from build123d import *

# Parameters (mm, degrees)
SKETCH1_W           = 280
SKETCH1_H           = 215
BOSS_EXTRUDE1_DEPTH = 10.6
FILLET1_R           = 18
CUT_EXTRUDE1_DEPTH  = 177.829324491
SKETCH3_R           = 1.6
SKETCH3_R_2         = 3.15
SKETCH3_R_3         = 1.7
SKETCH3_R_4         = 1.55
SKETCH3_R_5         = 2
CUT_EXTRUDE2_DEPTH  = 177.829324491


with BuildPart() as part:
    # Sketch1 → Boss-Extrude1 (new body)
    with BuildSketch(Plane(origin=(0, 0, 0), x_dir=(1, 0, 0), z_dir=(0, 1, 0))):
        Rectangle(SKETCH1_W, SKETCH1_H)
    extrude(amount=BOSS_EXTRUDE1_DEPTH)

    # Fillet1
    fillet1_edges = [part.edges().sort_by_distance(p)[0] for p in [
        (-140, 5.3, -107.5),
        (140, 5.3, -107.5),
        (140, 5.3, 107.5),
        (-140, 5.3, 107.5),
    ]]
    fillet(fillet1_edges, radius=FILLET1_R)

    # Sketch2 → Cut-Extrude1 (cut, through all)
    with BuildSketch(Plane(origin=(0, 10.6, 0), x_dir=(1, 0, 0), z_dir=(0, 1, 0))):
        with BuildLine():
            Line((-123.3, -36.5), (-123.3, 36.5))
            ThreePointArc((-123.3, 36.5), (-113.3, 46.5), (-103.3, 36.5))
            Line((-103.3, 36.5), (-103.3, -36.5))
            ThreePointArc((-103.3, -36.5), (-113.3, -46.5), (-123.3, -36.5))
        make_face()
    extrude(amount=-CUT_EXTRUDE1_DEPTH, mode=Mode.SUBTRACT)

    # Sketch3 → Cut-Extrude2 (cut, through all)
    with BuildSketch(Plane(origin=(0, 10.6, 0), x_dir=(1, 0, 0), z_dir=(0, 1, 0))):
        with Locations(Location((-131.75, -27.9, 0), (0, 0, 270))):
            Circle(SKETCH3_R)
        with Locations(Location((-131.75, 30.1, 0), (0, 0, 270))):
            Circle(SKETCH3_R)
        with Locations(Location((-70.6, 20, 0), (0, 0, 270))):
            Circle(SKETCH3_R_2)
        with Locations(Location((-70.6, 0, 0), (0, 0, 270))):
            Circle(SKETCH3_R_3)
        with Locations(Location((-28.3, -10.442748969, 0), (0, 0, 270))):
            Circle(SKETCH3_R)
        with Locations(Location((-37.3, -10.442748969, 0), (0, 0, 270))):
            Circle(SKETCH3_R)
        with Locations(Location((-37.3, 2.5, 0), (0, 0, 270))):
            Circle(SKETCH3_R_4)
        with Locations(Location((-37.3, 20, 0), (0, 0, 270))):
            Circle(SKETCH3_R)
        with Locations(Location((-37.3, 37.5, 0), (0, 0, 270))):
            Circle(SKETCH3_R_4)
        with Locations(Location((-28.3, 50.442748969, 0), (0, 0, 270))):
            Circle(SKETCH3_R)
        with Locations(Location((-37.3, 50.442748969, 0), (0, 0, 270))):
            Circle(SKETCH3_R)
        with Locations(Location((46.6, -4.8, 0), (0, 0, 270))):
            Circle(SKETCH3_R)
        with Locations(Location((46.6, 44.8, 0), (0, 0, 270))):
            Circle(SKETCH3_R)
        with Locations(Location((-70.6, 39.2, 0), (0, 0, 270))):
            Circle(SKETCH3_R_3)
        with Locations(Location((53.7, 44.8, 0), (0, 0, 270))):
            Circle(SKETCH3_R)
        with Locations(Location((53.7, -4.8, 0), (0, 0, 270))):
            Circle(SKETCH3_R)
        with Locations(Location((-39.5, -35, 0), (0, 0, 270))):
            Circle(SKETCH3_R_5)
        with Locations(Location((-14.5, -35, 0), (0, 0, 270))):
            Circle(SKETCH3_R_5)
        with Locations(Location((-39.5, -65, 0), (0, 0, 270))):
            Circle(SKETCH3_R_5)
        with Locations(Location((-14.5, -65, 0), (0, 0, 270))):
            Circle(SKETCH3_R_5)
        with Locations(Location((94.5, -35, 0), (0, 0, 270))):
            Circle(SKETCH3_R_5)
        with Locations(Location((119.5, -35, 0), (0, 0, 270))):
            Circle(SKETCH3_R_5)
        with Locations(Location((94.5, -65, 0), (0, 0, 270))):
            Circle(SKETCH3_R_5)
        with Locations(Location((119.5, -65, 0), (0, 0, 270))):
            Circle(SKETCH3_R_5)
    extrude(amount=-CUT_EXTRUDE2_DEPTH, mode=Mode.SUBTRACT)


solid = part.part
Read the model definition and answer for the solid it produces. Units are mm, in the model's axes. A direction names the side the tool comes from. Coordinates: 2 decimals unless noted, no trailing zeros. Loops run counter-clockwise (first coordinate to the right, second up) from the corner with the lowest first, then second, coordinate; pieces in that order, holes last. Notation, with made-up numbers: (55, 54.5) - (87, 54.5) arc R17 cw to (87, 82.5) - close; hole circle Ø5 at (31, 74). An arc over 180 degrees is marked (long way). Answer in a Markdown table with one row per item.
Q1. Find section C-C on y = 4.5. Count the separate pieces of the cut face and the enclosed holes in it, plus the area to 3 significant figures.
Here are the results:
| item | result |
|---|---|
| separate pieces | 1 |
| enclosed holes | 25 |
| area | 57,900 mm^2 |
Q2. Given P1, Ø3.5, axis at x = -14.5, z = 65, coming from the +Y side, flat-ended and moving along its own axis, determine where the tip first touches the part or whether it passes through.
Here are the results:
| item | result |
|---|---|
| P1 | passes through |
Q3. Find section A-A on z = 22. Write down the section's boundary in (x, y), plus the area to 3 significant figures.
Here are the results:
| item | result |
|---|---|
| outline | (-140, 0) - (-123.3, 0) - (-123.3, 10.6) - (-140, 10.6) - close; (-103.3, 0) - (140, 0) - (140, 10.6) - (-103.3, 10.6) - close |
| area | 2,760 mm^2 |
Q4. Straight lines are drawn through the part: line 1 along X through (y, z) = (7.75, 35); line 2 along X through (y, z) = (6.75, 4.8); line 3 along X through (y, z) = (7.5, 10). For each, find the intervals that lie inside material, in ascending order. Write a range as [from, to].
Here are the results:
| item | result |
|---|---|
| line 1 | x = [-140, -123.3], [-103.3, -41.5], [-37.5, -16.5], [-12.5, 92.5], [96.5, 117.5], [121.5, 140] |
| line 2 | x = [-140, -123.3], [-103.3, 45], [48.2, 52.1], [55.3, 140] |
| line 3 | x = [-140, -123.3], [-103.3, -38.84], [-35.76, -29.84], [-26.76, 140] |
Q5. For faces 1 (the cylindrical face through (-134.867, 5.374, 102.087)), 2 (the flat face through (-123.3, 5, 1)), determine the directions among +Z, -Z, +X, -X, +Y, -Y from which every point of the face is accessible in a straight line to the end or side of a thin tool.
Here are the results:
| item | result |
|---|---|
| face 1 | +Z, -X, +Y, -Y |
| face 2 | +Y, -Y |
Q6. The mould has two halves that part along Z. Classify faces 3 (the flat face through (-2, 10.6, -2)), 4 (the cylindrical face through (-67.477, 5.374, -20.41)), 5 (the cylindrical face through (-134.867, 5.374, -102.087)): pulls with the +Z half, pulls with the -Z half, needs draft (parallel to the pull), parting line crosses it, or undercut.
Here are the results:
| item | result |
|---|---|
| face 3 | needs draft |
| face 4 | undercut |
| face 5 | pulls with the -Z half |
Q7. Find section B-B on x = -113.3. Write down the section's boundary in (y, z), plus the area to 3 significant figures.
Here are the results:
| item | result |
|---|---|
| outline | (0, -107.5) - (10.6, -107.5) - (10.6, -46.5) - (0, -46.5) - close; (0, 46.5) - (10.6, 46.5) - (10.6, 107.5) - (0, 107.5) - close |
| area | 1,290 mm^2 |
